Geometry check sheet. Reference: the model listing, model coordinates, mm. Face numbers are marked on the shaded views. A direction names the side the tool comes from. Coordinates: 2 decimals unless noted, no trailing zeros. Order: outer loops, then holes, each group sorted by start corner. A loop starts at its lowest first (then second) coordinate and runs counter-clockwise, first axis right, second up. Notation, with made-up numbers: (44, 12) - (51, 12) arc R32 ccw to (51, 51) - close; hole circle Ø2 at (36, 3). An arc over 180 degrees is marked (long way). Return JSON: item names as keys, results as strings. Group by question number.
Item 1: Tool access check on the marked faces 5, 6 and 7. Record the directions out of +Z, -Z, +X, -X, +Y, -Y that give a thin tool (end or side, any length) a straight path to the whole face; none if there is none.
Item 2: Section check C-C on x = -42.25. Enter the section's corners in (y, z).
Item 3: Scan lines: probe 1 along X at (y, z) = (-4.5, 5); probe 2 along Z at (x, y) = (-39.75, 1); probe 3 along X at (y, z) = (-1, 6.5). Record each from-to range of solid material in increasing order.
Item 4: Draft check along X on the marked faces 1, 2, 3 and 4. Enter one of: pulls with the +X half, pulls with the -X half, needs draft (parallel to the pull), parting line crosses it, or undercut.
Item 5: Gauge pin test, flat end, axial feed: pin 1 (0.6 mm diameter, centred on x = -35.5, z = 7, fed in from -Y). Record the tip position at first contact, or that the pin passes through.
Item 6: Section check A-A on y = -6.25. Enter the section's corners in (x, z), then the cut area to 3 significant figures.
Item 7: Section check B-B on z = 1.75. Enter the section's corners in (x, y).
Item 8: Section check D-D on x = -20.75. Enter the section's corners in (y, z), then the cut area to 3 significant figures.
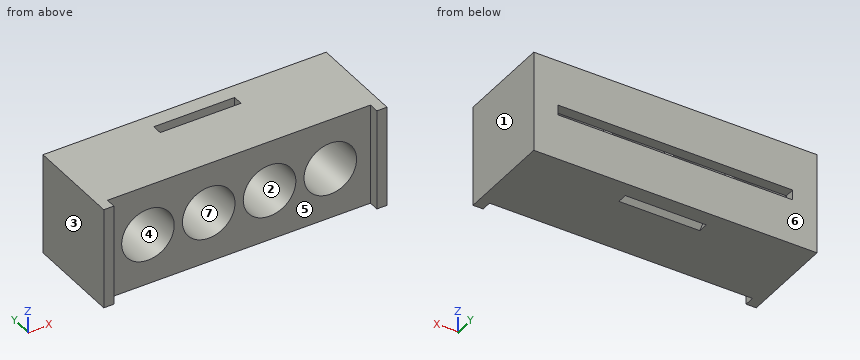
from build123d import *

# Parameters (mm, degrees)
SKICA1_W                 = 28
SKICA1_H                 = 8.5
P_IDAT_VYSUNUT_M1_DEPTH  = 10
SKICA3_R                 = 2.6
ODEBRAT_VYSUNUT_M2_DEPTH = 7.5
SKICA4_W                 = 23.2
SKICA4_H                 = 1
ODEBRAT_VYSUNUT_M3_DEPTH = 1
SKICA5_W                 = 1
SKICA5_H                 = 10
P_IDAT_VYSUNUT_M2_DEPTH  = 1
ODEBRAT_START            = -10
ODEBRAT_VYSUNUT_M5_DEPTH = 8


with BuildPart() as part:
    # Skica1 → Přidat vysunutím1 (new body)
    with BuildSketch(Plane.XY):
        with Locations((-32.656744291, -2.464704976)):
            Rectangle(SKICA1_W, SKICA1_H)
    extrude(amount=P_IDAT_VYSUNUT_M1_DEPTH)

    # Skica3 → Odebrat vysunutím2 (cut)
    with BuildSketch(Plane(origin=(0, -6.714704976, 0), x_dir=(-1, 0, 0), z_dir=(0, -1, 0))):
        with Locations((41.656744291, -5)):
            Circle(SKICA3_R)
        with Locations((35.646744291, -5)):
            Circle(SKICA3_R)
        with Locations((29.636744291, -5)):
            Circle(SKICA3_R)
        with Locations((23.626744291, -5)):
            Circle(SKICA3_R)
    extrude(amount=-ODEBRAT_VYSUNUT_M2_DEPTH, mode=Mode.SUBTRACT)

    # Skica4 → Odebrat vysunutím3 (cut)
    with BuildSketch(Plane(origin=(0, 1.785295024, 0), x_dir=(1, 0, 0), z_dir=(0, 1, 0))):
        with Locations((-32.656744291, -5)):
            Rectangle(SKICA4_W, SKICA4_H)
    extrude(amount=-ODEBRAT_VYSUNUT_M3_DEPTH, mode=Mode.SUBTRACT)

    # Skica5 → Přidat vysunutím2 (add)
    with BuildSketch(Plane(origin=(0, -6.714704976, 0), x_dir=(-1, 0, 0), z_dir=(0, -1, 0))):
        with Locations((46.156744291, -5)):
            Rectangle(SKICA5_W, SKICA5_H)
        with Locations((19.156744291, -5)):
            Rectangle(SKICA5_W, SKICA5_H)
    extrude(amount=P_IDAT_VYSUNUT_M2_DEPTH)

    # Skica9 → Odebrat vysunutím5 (cut)
    with BuildSketch(Plane(origin=(-18.656744291, 0, 0), x_dir=(0, 0, -1), z_dir=(1, 0, 0)).offset(ODEBRAT_START)):
        Polygon((-10, 0.285295024), (-9, 0.285295024), (-10, -0.714704976), align=None)
        Polygon((0, 0.285295024), (-1, 0.285295024), (0, -0.714704976), align=None)
    extrude(amount=-ODEBRAT_VYSUNUT_M5_DEPTH, mode=Mode.SUBTRACT)


solid = part.part
Computed:
{
 "1": {"face 5": "+Z, -Z, -Y", "face 6": "+Z, -Z, +X, -X, +Y", "face 7": "-Y"},
 "2": {"outline": "(-6.71, 0) - (1.79, 0) - (1.79, 4.5) - (0.79, 4.5) - (0.79, 2.47) - (-6.71, 2.47) - close; (-6.71, 7.53) - (0.79, 7.53) - (0.79, 5.5) - (1.79, 5.5) - (1.79, 10) - (-6.71, 10) - close"},
 "3": {"probe 1": "x = -46.66 to -44.26, -39.06 to -38.25, -33.05 to -32.24, -27.04 to -26.23, -21.03 to -18.66", "probe 2": "z = 0 to 4.5, 5.5 to 10", "probe 3": "x = -46.66 to -43.78, -39.53 to -37.77, -33.52 to -31.76, -27.51 to -25.75, -21.5 to -18.66"},
 "4": {"face 1": "pulls with the +X half", "face 2": "undercut", "face 3": "pulls with the -X half", "face 4": "undercut"},
 "5": {"pin 1": "stops at y = 0.79"},
 "6": {"outline": "(-46.66, 0) - (-18.66, 0) - (-18.66, 10) - (-46.66, 10) - close; hole circle Ø5.2 at (-41.66, 5); hole circle Ø5.2 at (-35.65, 5); hole circle Ø5.2 at (-29.64, 5); hole circle Ø5.2 at (-23.63, 5)", "area": "195 mm²"},
 "7": {"outline": "(-46.66, -7.71) - (-45.66, -7.71) - (-45.66, -6.71) - (-19.66, -6.71) - (-19.66, -7.71) - (-18.66, -7.71) - (-18.66, 1.79) - (-46.66, 1.79) - close"},
 "8": {"outline": "(-6.71, 0) - (1.79, 0) - (1.79, 10) - (-6.71, 10) - close", "area": "85.0 mm²"}
}
